Source: CAD feature listing. Evaluate the final solid. Frame: model axes, mm. Give positions to 0.01 mm unless a question says otherwise; leave off trailing zeros. Write each loop counter-clockwise with the first axis right and the second up, starting at its lowest first coordinate (ties: lowest second). Pieces come first, ordered by that corner, then holes. Notation, with made-up numbers: (4, 60.5) -> (39, 60.5) arc R18 ccw to (39, 84.5) -> close; hole circle Ø7 at (88.25, -31). An arc over 180 degrees is marked (long way). Write item = value, one per line.
from build123d import *

# Parameters (mm, degrees)
F1_DEPTH = 3


with BuildPart() as f1:
    # F0 (on Top) → F1 (new body)
    with BuildSketch(Plane.XY):
        with BuildLine():
            Line((-5.75, 385.5), (-5.75, 399.95867))
            ThreePointArc((-5.75, 399.95867), (-69.459271, 393.923101), (-131.390689, 377.804826))
            Line((-131.390689, 377.804826), (-126.445533, 364.218121))
            Line((-126.445533, 364.218121), (-137.251998, 360.284889))
            Line((-137.251998, 360.284889), (-142.197154, 373.871595))
            ThreePointArc((-142.197154, 373.871595), (-200, 346.410162), (-252.683722, 310.082145))
            Line((-252.683722, 310.082145), (-243.389868, 299.006162))
            Line((-243.389868, 299.006162), (-252.199379, 291.614104))
            Line((-252.199379, 291.614104), (-261.493233, 302.690088))
            ThreePointArc((-261.493233, 302.690088), (-306.417777, 257.115044), (-343.499368, 204.958981))
            Line((-343.499368, 204.958981), (-330.977793, 197.729646))
            Line((-330.977793, 197.729646), (-336.727793, 187.770354))
            Line((-336.727793, 187.770354), (-349.249368, 194.999689))
            ThreePointArc((-349.249368, 194.999689), (-375.877048, 136.808057), (-392.883922, 75.114739))
            Line((-392.883922, 75.114739), (-378.644912, 72.604017))
            Line((-378.644912, 72.604017), (-380.641866, 61.278728))
            Line((-380.641866, 61.278728), (-394.880876, 63.78945))
            ThreePointArc((-394.880876, 63.78945), (-400, 0), (-394.880876, -63.78945))
            Line((-394.880876, -63.78945), (-380.641866, -61.278728))
            Line((-380.641866, -61.278728), (-378.644912, -72.604017))
            Line((-378.644912, -72.604017), (-392.883922, -75.114739))
            ThreePointArc((-392.883922, -75.114739), (-375.877048, -136.808057), (-349.249368, -194.999689))
            Line((-349.249368, -194.999689), (-336.727793, -187.770354))
            Line((-336.727793, -187.770354), (-330.977793, -197.729646))
            Line((-330.977793, -197.729646), (-343.499368, -204.958981))
            ThreePointArc((-343.499368, -204.958981), (-306.417777, -257.115044), (-261.493233, -302.690088))
            Line((-261.493233, -302.690088), (-252.199379, -291.614104))
            Line((-252.199379, -291.614104), (-243.389868, -299.006162))
            Line((-243.389868, -299.006162), (-252.683722, -310.082145))
            ThreePointArc((-252.683722, -310.082145), (-200, -346.410162), (-142.197154, -373.871595))
            Line((-142.197154, -373.871595), (-137.251998, -360.284889))
            Line((-137.251998, -360.284889), (-126.445533, -364.218121))
            Line((-126.445533, -364.218121), (-131.390689, -377.804826))
            ThreePointArc((-131.390689, -377.804826), (-69.459271, -393.923101), (-5.75, -399.95867))
            Line((-5.75, -399.95867), (-5.75, -385.5))
            Line((-5.75, -385.5), (5.75, -385.5))
            Line((5.75, -385.5), (5.75, -399.95867))
            ThreePointArc((5.75, -399.95867), (69.459271, -393.923101), (131.390689, -377.804826))
            Line((131.390689, -377.804826), (126.445533, -364.218121))
            Line((126.445533, -364.218121), (137.251998, -360.284889))
            Line((137.251998, -360.284889), (142.197154, -373.871595))
            ThreePointArc((142.197154, -373.871595), (200, -346.410162), (252.683722, -310.082145))
            Line((252.683722, -310.082145), (243.389868, -299.006162))
            Line((243.389868, -299.006162), (252.199379, -291.614104))
            Line((252.199379, -291.614104), (261.493233, -302.690088))
            ThreePointArc((261.493233, -302.690088), (306.417777, -257.115044), (343.499368, -204.958981))
            Line((343.499368, -204.958981), (330.977793, -197.729646))
            Line((330.977793, -197.729646), (336.727793, -187.770354))
            Line((336.727793, -187.770354), (349.249368, -194.999689))
            ThreePointArc((349.249368, -194.999689), (375.877048, -136.808057), (392.883922, -75.114739))
            Line((392.883922, -75.114739), (378.644912, -72.604017))
            Line((378.644912, -72.604017), (380.641866, -61.278728))
            Line((380.641866, -61.278728), (394.880876, -63.78945))
            ThreePointArc((394.880876, -63.78945), (400, 0), (394.880876, 63.78945))
            Line((394.880876, 63.78945), (380.641866, 61.278728))
            Line((380.641866, 61.278728), (378.644912, 72.604017))
            Line((378.644912, 72.604017), (392.883922, 75.114739))
            ThreePointArc((392.883922, 75.114739), (375.877048, 136.808057), (349.249368, 194.999689))
            Line((349.249368, 194.999689), (336.727793, 187.770354))
            Line((336.727793, 187.770354), (330.977793, 197.729646))
            Line((330.977793, 197.729646), (343.499368, 204.958981))
            ThreePointArc((343.499368, 204.958981), (306.417777, 257.115044), (261.493233, 302.690088))
            Line((261.493233, 302.690088), (252.199379, 291.614104))
            Line((252.199379, 291.614104), (243.389868, 299.006162))
            Line((243.389868, 299.006162), (252.683722, 310.082145))
            ThreePointArc((252.683722, 310.082145), (200, 346.410162), (142.197154, 373.871595))
            Line((142.197154, 373.871595), (137.251998, 360.284889))
            Line((137.251998, 360.284889), (126.445533, 364.218121))
            Line((126.445533, 364.218121), (131.390689, 377.804826))
            ThreePointArc((131.390689, 377.804826), (69.459271, 393.923101), (5.75, 399.95867))
            Line((5.75, 399.95867), (5.75, 385.5))
            Line((5.75, 385.5), (-5.75, 385.5))
        make_face()
    extrude(amount=F1_DEPTH)


solid = f1.part
1) Cut plane A-A (y = -147.5). Return the cut outline in (x, z).
Computed:
outline = (-371.81, 0) -> (371.81, 0) -> (371.81, 3) -> (-371.81, 3) -> close
2) Material intervals for L1, parallel to Y at x = 63.5, z = 0.8; L2, parallel to Y at x = -195, z = 1; L3, parallel to X at y = 11, z = 2.85, sorted ascending.
Computed:
L1 = -394.93 to 394.93
L2 = -349.25 to 349.25
L3 = -399.85 to 399.85
3) Contact query for flat-ended pins moving along their axis: pin 1 (1.5 mm diameter, centred on x = 1, z = 2, fed in from -Y); pin 2 (1.5 mm diameter, centred on x = -1.5, z = 1, fed in from +Y); pin 3 (1.5 mm diameter, centred on y = -68.5, z = 1, fed in from +X). Output: stop coordinate, or through.
Computed:
pin_1 = -385.5
pin_2 = 385.5
pin_3 = 379.5
4) Cut plane B-B (x = 85). Return the cut outline in (y, z).
Computed:
outline = (-390.86, 0) -> (390.86, 0) -> (390.86, 3) -> (-390.86, 3) -> close
